```python
from build123d import *

# Parameters (mm, degrees)
SKETCH_2_W                 = 130
SKETCH_2_H                 = 125
SKETCH_2_R                 = 6
EXTRUDE_1_DEPTH            = 65
HOLE_WIZARD_4_0_4_5_D      = 4
HOLE_WIZARD_M5_3_D         = 4.2
HOLE_WIZARD_M5_3_DEPTH     = 12
HOLE_WIZARD_M5_3_TIP       = 1.2618073
HOLE_WIZARD_4_0_4_9_D      = 4
HOLE_WIZARD_4_0_4_9_DEPTH  = 32.5
HOLE_WIZARD_4_0_4_9_TIP    = 1.201721238
HOLE_WIZARD_6_0_6_1_D      = 6
HOLE_WIZARD_6_0_6_1_DEPTH  = 42
HOLE_WIZARD_6_0_6_1_TIP    = 1.802581857
HOLE_WIZARD_M6_1_D         = 5
HOLE_WIZARD_M6_1_DEPTH     = 13
HOLE_WIZARD_M6_1_TIP       = 1.502151548
HOLE_WIZARD_4_0_4_11_D     = 4
HOLE_WIZARD_4_0_4_11_DEPTH = 85
HOLE_WIZARD_4_0_4_11_TIP   = 1.201721238
M10X1_0_1_D                = 9
M10X1_0_1_DEPTH            = 13
M10X1_0_1_TIP              = 2.703872786
HOLE_WIZARD_1_D            = 12
HOLE_WIZARD_1_DEPTH        = 65
HOLE_WIZARD_1_CBORE_D      = 21.3
HOLE_WIZARD_1_CBORE_DEPTH  = 1.97
HOLE_WIZARD_8_0_8_1_D      = 8
HOLE_WIZARD_8_0_8_1_DEPTH  = 15.5
HOLE_WIZARD_8_0_8_1_TIP    = 2.403442476
HOLE_WIZARD_M5_5_D         = 4.2
HOLE_WIZARD_M5_5_DEPTH     = 10
HOLE_WIZARD_M5_5_TIP       = 1.2618073
HOLE_WIZARD_6_0_6_2_D      = 6
HOLE_WIZARD_6_0_6_2_DEPTH  = 58.5
HOLE_WIZARD_6_0_6_2_TIP    = 1.802581857
HOLE_WIZARD_6_0_6_3_D      = 6
HOLE_WIZARD_6_0_6_3_DEPTH  = 90
HOLE_WIZARD_6_0_6_3_TIP    = 1.802581857
HOLE_WIZARD_M5_8_D         = 4.2
HOLE_WIZARD_M5_8_DEPTH     = 41.31
HOLE_WIZARD_M5_8_TIP       = 1.2618073
HOLE_WIZARD_6_0_6_4_D      = 6
M10X1_0_2_D                = 9
M10X1_0_2_DEPTH            = 13
M10X1_0_2_TIP              = 2.703872786


with BuildPart() as part:
    # 草图2 → 凸台-拉伸1 (new body)
    with BuildSketch(Plane(origin=(0, 0, 0), x_dir=(1, 0, 0), z_dir=(0, 1, 0))):
        Rectangle(SKETCH_2_W, SKETCH_2_H)
        with Locations((-55, 52.5)):
            Circle(SKETCH_2_R, mode=Mode.SUBTRACT)
        with Locations((55, 52.5)):
            Circle(SKETCH_2_R, mode=Mode.SUBTRACT)
        with Locations((55, -52.5)):
            Circle(SKETCH_2_R, mode=Mode.SUBTRACT)
        with Locations((-55, -52.5)):
            Circle(SKETCH_2_R, mode=Mode.SUBTRACT)
    extrude(amount=EXTRUDE_1_DEPTH)

    # Ø4.0 (4) 直径孔5 (through all)
    with Locations(Plane(origin=(-65, 38, -22.5), x_dir=(0, 0, -1), z_dir=(-1, 0, 0))):
        with Locations((0, 0)):
            Hole(HOLE_WIZARD_4_0_4_5_D / 2)

    # M5 螺纹孔3
    with Locations(Plane(origin=(65, 48.3, -4.65), x_dir=(0, 0, 1), z_dir=(1, 0, 0))):
        with Locations((0, 0), (-32.5, 0), (-31.75, 40.5), (-0.75, 40.5)):
            Hole(HOLE_WIZARD_M5_3_D / 2, depth=HOLE_WIZARD_M5_3_DEPTH)
            with Locations((0, 0, -(HOLE_WIZARD_M5_3_DEPTH + HOLE_WIZARD_M5_3_TIP / 2))):  # 118° drill point
                Cone(0, HOLE_WIZARD_M5_3_D / 2, HOLE_WIZARD_M5_3_TIP, mode=Mode.SUBTRACT)

    # Ø4.0 (4) 直径孔9
    with Locations(Plane(origin=(65, 20.5, -22.49541266), x_dir=(0, 0, 1), z_dir=(1, 0, 0))):
        with Locations((0, 0)):
            Hole(HOLE_WIZARD_4_0_4_9_D / 2, depth=HOLE_WIZARD_4_0_4_9_DEPTH)
            with Locations((0, 0, -(HOLE_WIZARD_4_0_4_9_DEPTH + HOLE_WIZARD_4_0_4_9_TIP / 2))):  # 118° drill point
                Cone(0, HOLE_WIZARD_4_0_4_9_D / 2, HOLE_WIZARD_4_0_4_9_TIP, mode=Mode.SUBTRACT)

    # Ø6.0 (6) 直径孔1
    with Locations(Plane(origin=(32.5, 20.5, -62.5), x_dir=(-1, 0, 0), z_dir=(0, 0, -1))):
        with Locations((0, 0)):
            Hole(HOLE_WIZARD_6_0_6_1_D / 2, depth=HOLE_WIZARD_6_0_6_1_DEPTH)
            with Locations((0, 0, -(HOLE_WIZARD_6_0_6_1_DEPTH + HOLE_WIZARD_6_0_6_1_TIP / 2))):  # 118° drill point
                Cone(0, HOLE_WIZARD_6_0_6_1_D / 2, HOLE_WIZARD_6_0_6_1_TIP, mode=Mode.SUBTRACT)

    # M6 螺纹孔1
    with Locations(Plane(origin=(-65, 52.5, -37), x_dir=(0, 0, -1), z_dir=(-1, 0, 0))):
        with Locations((0, 0), (-29, 0), (0, 29), (-29, 29)):
            Hole(HOLE_WIZARD_M6_1_D / 2, depth=HOLE_WIZARD_M6_1_DEPTH)
            with Locations((0, 0, -(HOLE_WIZARD_M6_1_DEPTH + HOLE_WIZARD_M6_1_TIP / 2))):  # 118° drill point
                Cone(0, HOLE_WIZARD_M6_1_D / 2, HOLE_WIZARD_M6_1_TIP, mode=Mode.SUBTRACT)

    # Ø4.0 (4) 直径孔11
    with Locations(Plane(origin=(-30, 38, 62.5), x_dir=(1, 0, 0), z_dir=(0, 0, 1))):
        with Locations((0, 0)):
            Hole(HOLE_WIZARD_4_0_4_11_D / 2, depth=HOLE_WIZARD_4_0_4_11_DEPTH)
            with Locations((0, 0, -(HOLE_WIZARD_4_0_4_11_DEPTH + HOLE_WIZARD_4_0_4_11_TIP / 2))):  # 118° drill point
                Cone(0, HOLE_WIZARD_4_0_4_11_D / 2, HOLE_WIZARD_4_0_4_11_TIP, mode=Mode.SUBTRACT)

    # M10x1.0 螺纹孔1
    with Locations(Plane(origin=(-30, 38, 62.5), x_dir=(1, 0, 0), z_dir=(0, 0, 1))):
        with Locations((0, 0)):
            Hole(M10X1_0_1_D / 2, depth=M10X1_0_1_DEPTH)
            with Locations((0, 0, -(M10X1_0_1_DEPTH + M10X1_0_1_TIP / 2))):  # 118° drill point
                Cone(0, M10X1_0_1_D / 2, M10X1_0_1_TIP, mode=Mode.SUBTRACT)

    # 孔1
    with Locations(Plane(origin=(-5, 65, 7.5), x_dir=(0, 0, 1), z_dir=(0, 1, 0))):
        with Locations((0, 0), (20, 40)):
            CounterBoreHole(HOLE_WIZARD_1_D / 2, HOLE_WIZARD_1_CBORE_D / 2, HOLE_WIZARD_1_CBORE_DEPTH, depth=HOLE_WIZARD_1_DEPTH)

    # Ø8.0 (8) 直径孔1
    with Locations(Plane(origin=(23, 0, -3.7), x_dir=(0, 0, -1), z_dir=(0, -1, 0))):
        with Locations((0, 0)):
            Hole(HOLE_WIZARD_8_0_8_1_D / 2, depth=HOLE_WIZARD_8_0_8_1_DEPTH)
            with Locations((0, 0, -(HOLE_WIZARD_8_0_8_1_DEPTH + HOLE_WIZARD_8_0_8_1_TIP / 2))):  # 118° drill point
                Cone(0, HOLE_WIZARD_8_0_8_1_D / 2, HOLE_WIZARD_8_0_8_1_TIP, mode=Mode.SUBTRACT)

    # M5 螺纹孔5
    with Locations(Plane(origin=(4.7, 36, -62.5), x_dir=(-1, 0, 0), z_dir=(0, 0, -1))):
        with Locations((0, 0), (-40.5, 0), (-40.5, -31), (0, -31)):
            Hole(HOLE_WIZARD_M5_5_D / 2, depth=HOLE_WIZARD_M5_5_DEPTH)
            with Locations((0, 0, -(HOLE_WIZARD_M5_5_DEPTH + HOLE_WIZARD_M5_5_TIP / 2))):  # 118° drill point
                Cone(0, HOLE_WIZARD_M5_5_D / 2, HOLE_WIZARD_M5_5_TIP, mode=Mode.SUBTRACT)

    # Ø6.0 (6) 直径孔2
    with Locations(Plane(origin=(23.7, 10.1, -62.5), x_dir=(-1, 0, 0), z_dir=(0, 0, -1))):
        with Locations((0, 0)):
            Hole(HOLE_WIZARD_6_0_6_2_D / 2, depth=HOLE_WIZARD_6_0_6_2_DEPTH)
            with Locations((0, 0, -(HOLE_WIZARD_6_0_6_2_DEPTH + HOLE_WIZARD_6_0_6_2_TIP / 2))):  # 118° drill point
                Cone(0, HOLE_WIZARD_6_0_6_2_D / 2, HOLE_WIZARD_6_0_6_2_TIP, mode=Mode.SUBTRACT)

    # Ø6.0 (6) 直径孔3
    with Locations(Plane(origin=(23.7, 30.9, -62.5), x_dir=(-1, 0, 0), z_dir=(0, 0, -1))):
        with Locations((0, 0)):
            Hole(HOLE_WIZARD_6_0_6_3_D / 2, depth=HOLE_WIZARD_6_0_6_3_DEPTH)
            with Locations((0, 0, -(HOLE_WIZARD_6_0_6_3_DEPTH + HOLE_WIZARD_6_0_6_3_TIP / 2))):  # 118° drill point
                Cone(0, HOLE_WIZARD_6_0_6_3_D / 2, HOLE_WIZARD_6_0_6_3_TIP, mode=Mode.SUBTRACT)

    # M5 螺纹孔8
    with Locations(Plane(origin=(65, 30.9, 28.70458734), x_dir=(0, 0, 1), z_dir=(1, 0, 0))):
        with Locations((0, 0)):
            Hole(HOLE_WIZARD_M5_8_D / 2, depth=HOLE_WIZARD_M5_8_DEPTH)
            with Locations((0, 0, -(HOLE_WIZARD_M5_8_DEPTH + HOLE_WIZARD_M5_8_TIP / 2))):  # 118° drill point
                Cone(0, HOLE_WIZARD_M5_8_D / 2, HOLE_WIZARD_M5_8_TIP, mode=Mode.SUBTRACT)

    # Ø6.0 (6) 直径孔4 (through all)
    with Locations(Plane(origin=(15, 20.5, -62.5), x_dir=(-1, 0, 0), z_dir=(0, 0, -1))):
        with Locations((0, 0)):
            Hole(HOLE_WIZARD_6_0_6_4_D / 2)

    # M10x1.0 螺纹孔2
    with Locations(Plane(origin=(15, 20.5, 62.5), x_dir=(1, 0, 0), z_dir=(0, 0, 1))):
        with Locations((0, 0)):
            Hole(M10X1_0_2_D / 2, depth=M10X1_0_2_DEPTH)
            with Locations((0, 0, -(M10X1_0_2_DEPTH + M10X1_0_2_TIP / 2))):  # 118° drill point
                Cone(0, M10X1_0_2_D / 2, M10X1_0_2_TIP, mode=Mode.SUBTRACT)


solid = part.part
```
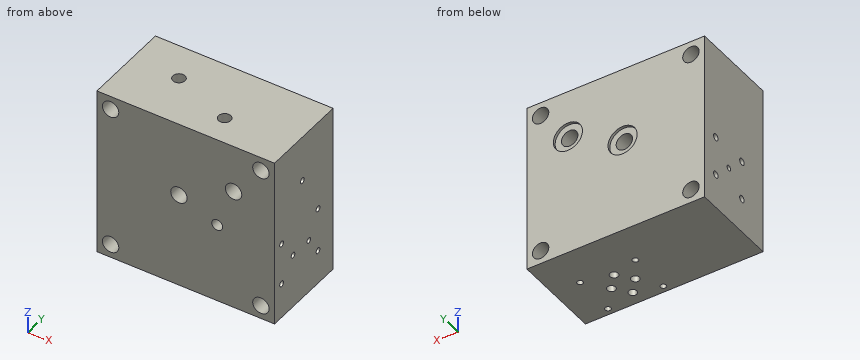
Geometry: final body of the model. Coordinates: model frame, mm. Round coordinates to 2 decimals unless told otherwise and drop trailing zeros. Loops run counter-clockwise (first coordinate to the right, second up) from the corner with the lowest first, then second, coordinate; pieces in that order, holes last. Notation, with made-up numbers: (55, 19) -> (102, 19) arc R29 ccw to (102, 54) -> close; hole circle Ø7 at (27, 80.5). An arc over 180 degrees is marked (long way). Use one line per item in the form item = value.
Item 1: Material intervals for probe 1 along Y at (x, z) = (23.7, -22.5); probe 2 along Y at (x, z) = (23.7, -41.5); probe 3 along Z at (x, y) = (50, 20), sorted ascending.
Evaluation:
probe_1 = 0 to 7.1, 13.1 to 27.9, 33.9 to 36, 40 to 65
probe_2 = 0 to 7.1, 13.1 to 27.9, 33.9 to 65
probe_3 = -62.5 to -55.82, -49.18 to -24.43, -20.56 to 49.18, 55.82 to 62.5
Item 2: Cut plane A-A on z = 5.5. Output: boundary loops of the cut face in (x, y), then the cut area to 3 significant figures.
Evaluation:
outline = (-65, 0) -> (-10.66, 0) -> (-10.66, 63.03) -> (-15.46, 63.03) -> (-15.46, 65) -> (-65, 65) -> close; (0.66, 0) -> (65, 0) -> (65, 65) -> (5.46, 65) -> (5.46, 63.03) -> (0.66, 63.03) -> close; hole circle Ø4 at (-30, 38); hole circle Ø6 at (15, 20.5); hole circle Ø6 at (23.7, 30.9)
area = 7,630 mm2
Item 3: Contact query for flat-ended pins moving along their axis: pin 1 Ø3 at (x, y) = (-30, 38) entering from +Z; pin 2 Ø15.5 at (x, z) = (-5, 7.5) entering from -Y; pin 3 Ø9.5 at (x, z) = (-55, -52.5) entering from -Y; pin 4 Ø3.5 at (y, z) = (30.9, 28.7) entering from +X. Output: stop coordinate, or through.
Evaluation:
pin_1 = -23.82
pin_2 = 0
pin_3 = through
pin_4 = 23.48
Item 4: Cut plane B-B on x = 15.5. Give the number of separate pieces and of enclosed holes in the cut face, then the cut area to 3 significant figures.
Evaluation:
separate_pieces = 2
enclosed_holes = 1
area = 7,330 mm2
